```python
from build123d import *

# Parameters (mm, degrees)
SKETCH2_R               = 1.5
BOSS_EXTRUDE1_DEPTH     = 3
SKETCH5_W               = 5
SKETCH5_H               = 15
BOSS_EXTRUDE3_DEPTH     = 15
CUT_EXTRUDE1_DEPTH      = 118.579760163
CUT_EXTRUDE1_DEPTH_BACK = 118.579760163
SKETCH6_R               = 5
FILLET1_R               = 7.5
FILLET2_R               = 2
SKETCH7_R               = 2.5
SKETCH7_R_2             = 1
BOSS_EXTRUDE4_DEPTH     = 15
CUT_EXTRUDE2_DEPTH      = 106.943381105
CUT_EXTRUDE2_DEPTH_BACK = 106.943381105
BOSS_EXTRUDE5_DEPTH     = 3


with BuildPart() as part:
    # Sketch2 → Boss-Extrude1 (new body)
    with BuildSketch(Plane(origin=(0, 0, 0), x_dir=(1, 0, 0), z_dir=(0, 1, 0))):
        Polygon((30, 0), (-30, 0), (-30, 56.5), (-21.111111111, 68.5), (-21.111111111, 71.5), (-30, 83.5), (-30, 86.5), (-20, 100), (20, 100), (30, 86.5), (30, 83.5), (21.111111111, 71.5), (21.111111111, 68.5), (30, 56.5), align=None)
        with Locations(Location((-20, 85, 0), (0, 0, 270))):
            Circle(SKETCH2_R, mode=Mode.SUBTRACT)
        with Locations(Location((20, 85, 0), (0, 0, 90))):
            Circle(SKETCH2_R, mode=Mode.SUBTRACT)
    extrude(amount=BOSS_EXTRUDE1_DEPTH)

    # Sketch5 → Boss-Extrude3 (add)
    with BuildSketch(Plane.XZ):
        with Locations((-27.5, -17)):
            Rectangle(SKETCH5_W, SKETCH5_H)
        with Locations((27.5, -17)):
            Rectangle(SKETCH5_W, SKETCH5_H)
    extrude(amount=BOSS_EXTRUDE3_DEPTH)

    # Sketch6 → Cut-Extrude1 (cut, two sides: drawn at the far end of the back side and taken through both)
    with BuildSketch(Plane.ZY.offset(30).offset(-CUT_EXTRUDE1_DEPTH_BACK)):
        with Locations((-17, -7.5)):
            Circle(SKETCH6_R)
    extrude(amount=CUT_EXTRUDE1_DEPTH + CUT_EXTRUDE1_DEPTH_BACK, mode=Mode.SUBTRACT)

    # Fillet1
    fillet1_edges = [part.edges().sort_by_distance(p)[0] for p in [
        (27.5, -15, -9.5),
        (27.5, -15, -24.5),
        (-27.5, -15, -24.5),
        (-27.5, -15, -9.5),
    ]]
    fillet(fillet1_edges, radius=FILLET1_R - 0.0001)  # a hair under: the kernel refuses the full size

    # Fillet2
    fillet2_edges = [part.edges().sort_by_distance(p)[0] for p in [
        (-27.5, 0, -24.5),
        (-25, 0, -17),
        (-27.5, 0, -9.5),
        (25, 0, -17),
        (27.5, 0, -24.5),
        (27.5, 0, -9.5),
    ]]
    fillet(fillet2_edges, radius=FILLET2_R)

    # Sketch7 → Boss-Extrude4 (add)
    # profile 1 of 4: a face of its own
    with BuildSketch(Plane(origin=(0, 3, 0), x_dir=(1, 0, 0), z_dir=(0, 1, 0))):
        with Locations(Location((25, 5, 0), (0, 0, 270))):
            Circle(SKETCH7_R)
        with Locations(Location((25, 5, 0), (0, 0, 270))):
            Circle(SKETCH7_R_2, mode=Mode.SUBTRACT)
    # profile 2 of 4: a face of its own
    with BuildSketch(Plane(origin=(0, 3, 0), x_dir=(1, 0, 0), z_dir=(0, 1, 0))):
        with Locations(Location((-25, 5, 0), (0, 0, 90))):
            Circle(SKETCH7_R)
        with Locations(Location((-25, 5, 0), (0, 0, 90))):
            Circle(SKETCH7_R_2, mode=Mode.SUBTRACT)
    # profile 3 of 4: a face of its own
    with BuildSketch(Plane(origin=(0, 3, 0), x_dir=(1, 0, 0), z_dir=(0, 1, 0))):
        with Locations(Location((17.481371253, 95, 0), (0, 0, 270))):
            Circle(SKETCH7_R)
        with Locations(Location((17.481371253, 95, 0), (0, 0, 270))):
            Circle(SKETCH7_R_2, mode=Mode.SUBTRACT)
    # profile 4 of 4: a face of its own
    with BuildSketch(Plane(origin=(0, 3, 0), x_dir=(1, 0, 0), z_dir=(0, 1, 0))):
        with Locations(Location((-17.481371253, 95, 0), (0, 0, 90))):
            Circle(SKETCH7_R)
        with Locations(Location((-17.481371253, 95, 0), (0, 0, 90))):
            Circle(SKETCH7_R_2, mode=Mode.SUBTRACT)
    extrude(amount=BOSS_EXTRUDE4_DEPTH)

    # Sketch8 → Cut-Extrude2 (cut, two sides: drawn at the far end of the back side and taken through both)
    with BuildSketch(Plane.XZ.offset(-CUT_EXTRUDE2_DEPTH_BACK)):
        Polygon((-18, -5), (-18, -31.5), (-25, -31.5), (-25, -54.849851192), (-15.555279985, -67.600223212), (-15.555279985, -72.399776788), (-10, -79.899404767), (-10, -88.299553575), (-5.036706352, -95), (5.036706352, -95), (10, -88.299553575), (10, -79.899404767), (15.555279985, -72.399776788), (15.555279985, -67.600223212), (25, -54.849851192), (25, -31.5), (18, -31.5), (18, -5), align=None)
    extrude(amount=CUT_EXTRUDE2_DEPTH + CUT_EXTRUDE2_DEPTH_BACK, mode=Mode.SUBTRACT)

    # Sketch9 → Boss-Extrude5 (add)
    with BuildSketch(Plane(origin=(0, 0, 0), x_dir=(1, 0, 0), z_dir=(0, 1, 0))):
        Polygon((-25, 50), (-5, 50), (-5, 0), (5, 0), (5, 50), (25, 50), (25, 54.849851192), (21.185074957, 60), (-21.185074957, 60), (-25, 54.849851192), align=None)
    extrude(amount=BOSS_EXTRUDE5_DEPTH)


solid = part.part
```
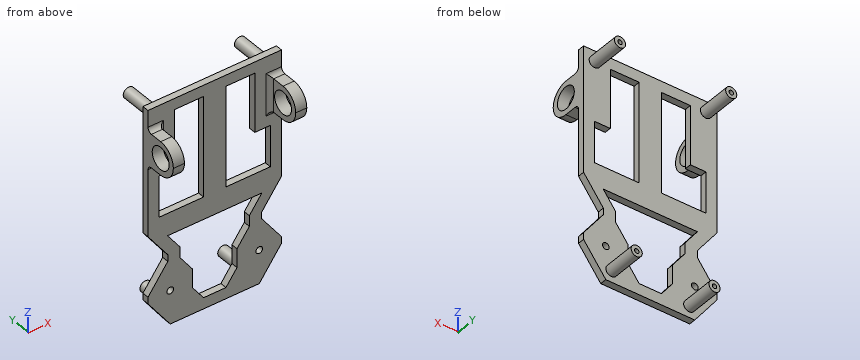
Geometry: final body of the model. Coordinates: model frame, mm. Round coordinates to 2 decimals unless told otherwise and drop trailing zeros. Order: outer loops, then holes, each group sorted by start corner. A loop starts at its lowest first (then second) coordinate and runs counter-clockwise, first axis right, second up. Notation, with made-up numbers: (-11.75, 0) -> (1.25, 0) arc R11 cw to (1.25, 17) -> close; hole circle Ø4 at (24.25, 79.25). An arc over 180 degrees is marked (long way). Use one line per item in the form item = value. Start each with the question number.
1. Cut plane B-B (y = 5.5). Return the cut outline in (x, z).
2. Pin query (flat end, axial travel): pin 1 Ø2.5 at (x, y) = (27.5, -6) entering from -Z; pin 2 Ø1.5 at (y, z) = (2, -71) entering from +X; pin 3 Ø3.5 at (y, z) = (1.5, -70.5) entering from -X; pin 4 Ø10 at (x, z) = (15, -40.5) entering from +Y. Return the tip coordinate at first contact, or that it passes through.
3. Line query: probe 1 along Z at (x, y) = (-25, 9); probe 2 along Y at (x, z) = (-27.6, -17); probe 3 along Y at (x, z) = (-9.5, -55.5). Output: solid intervals per line, ascending.
4. Cut plane D-D (z = -65.5). Return the cut outline in (x, y).
5. Cut plane A-A (x = 3). Return the cut outline in (y, z).
6. Cut plane C-C (y = -3.5). Return the cut outline in (x, z).
Solution:
q1.outline = circle Ø5 at (-25, -5); circle Ø5 at (-17.48, -95); circle Ø5 at (17.48, -95); circle Ø5 at (25, -5); hole circle Ø2 at (-25, -5); hole circle Ø2 at (-17.48, -95); hole circle Ø2 at (17.48, -95); hole circle Ø2 at (25, -5)
q2.pin_1 = -24.5
q2.pin_2 = 21.3
q2.pin_3 = -21.67
q2.pin_4 = through
q3.probe_1 = -7.5 to -6, -4 to -2.5
q3.probe_2 = -15 to -12.5, -2.5 to 3
q3.probe_3 = 0 to 3
q4.outline = (-23.33, 0) -> (-17.11, 0) -> (-17.11, 3) -> (-23.33, 3) -> close; (17.11, 0) -> (23.33, 0) -> (23.33, 3) -> (17.11, 3) -> close
q5.outline = (0, -100) -> (3, -100) -> (3, -95) -> (0, -95) -> close; (0, -60) -> (3, -60) -> (3, 0) -> (0, 0) -> close
q6.outline = (-30, -24.5) -> (-25, -24.5) -> (-25, -20) -> (-30, -20) -> close; (-30, -14) -> (-25, -14) -> (-25, -9.5) -> (-30, -9.5) -> close; (25, -24.5) -> (30, -24.5) -> (30, -20) -> (25, -20) -> close; (25, -14) -> (30, -14) -> (30, -9.5) -> (25, -9.5) -> close
